The listing builds one solid part. Answer for the finished solid, in the listing's coordinates (mm). Round coordinates to 2 decimals unless told otherwise and drop trailing zeros.
(1) Find the intervals of material crossed by probe 1 along X at (y, z) = (72.5, 6.75); probe 2 along Y at (x, z) = (183.5, 1.5); probe 3 along Y at (x, z) = (10, 5), in increasing order.
(2) This flat-tipped pin is pushed along its axis until it touches: pin 1 Ø7 at (x, y) = (10, 20) entering from -Z. Where does it stop, or does it pass through?
(3) The mould has two halves that part along Y. Classify faces 1 (the face through (247, 51, 7.5)), 2 (the face through (7.05, 22.7, 3.8)), 3 (the face through (9.133, 76.095, 3.802)): +Y half, -Y half, draft (parallel to the pull), parting line (faces both ways), or undercut.
from build123d import *

# Parameters (mm, degrees)
SKETCH2_W           = 500
SKETCH2_H           = 100
BOSS_EXTRUDE1_DEPTH = 7.5
SKETCH8_R           = 3
CUT_EXTRUDE2_DEPTH  = 510.957106039
SKETCH9_R           = 3
SKETCH9_R_2         = 2
CUT_EXTRUDE3_DEPTH  = 510.957106039
SKETCH11_R          = 4
CUT_EXTRUDE4_DEPTH  = 510.957106039


with BuildPart() as part:
    # Sketch2 → Boss-Extrude1 (new body)
    with BuildSketch(Plane.XY):
        with Locations((250, 50)):
            Rectangle(SKETCH2_W, SKETCH2_H)
    extrude(amount=BOSS_EXTRUDE1_DEPTH)

    # Sketch8 → Cut-Extrude2 (cut, through all)
    with BuildSketch(Plane.XY.offset(7.5)):
        with Locations((183.5, 23.5)):
            Circle(SKETCH8_R)
        with Locations((183.5, 72)):
            Circle(SKETCH8_R)
        with Locations((232, 72)):
            Circle(SKETCH8_R)
        with Locations((232, 23.5)):
            Circle(SKETCH8_R)
    extrude(amount=-CUT_EXTRUDE2_DEPTH, mode=Mode.SUBTRACT)

    # Sketch9 → Cut-Extrude3 (cut, through all)
    with BuildSketch(Plane.XY.offset(7.5)):
        with Locations((125, 48.5)):
            Circle(SKETCH9_R)
        with Locations((135.5, 48.5)):
            Circle(SKETCH9_R_2)
        with Locations((114.5, 48.5)):
            Circle(SKETCH9_R_2)
        with Locations((378, 48.5)):
            Circle(SKETCH9_R)
        with Locations((387.5, 48.5)):
            Circle(SKETCH9_R_2)
        with Locations((364.5, 48.5)):
            Circle(SKETCH9_R_2)
    extrude(amount=-CUT_EXTRUDE3_DEPTH, mode=Mode.SUBTRACT)

    # Sketch11 → Cut-Extrude4 (cut, through all)
    with BuildSketch(Plane.XY.offset(7.5)):
        with Locations((10, 80)):
            Circle(SKETCH11_R)
        with Locations((10, 20)):
            Circle(SKETCH11_R)
        with Locations((490, 20)):
            Circle(SKETCH11_R)
        with Locations((490, 80)):
            Circle(SKETCH11_R)
    extrude(amount=-CUT_EXTRUDE4_DEPTH, mode=Mode.SUBTRACT)


solid = part.part
Solutions:
1. probe 1: x = 0 to 180.54, 186.46 to 229.04, 234.96 to 500
1. probe 2: y = 0 to 20.5, 26.5 to 69, 75 to 100
1. probe 3: y = 0 to 16, 24 to 76, 84 to 100
2. pin 1: passes through
3. face 1: draft
3. face 2: undercut
3. face 3: undercut
